The listing builds one solid part. Answer for the finished solid, in the listing's coordinates (mm). A direction names the side the tool comes from. Give positions to 0.01 mm unless a question says otherwise; leave off trailing zeros. Order: outer loops, then holes, each group sorted by start corner. A loop starts at its lowest first (then second) coordinate and runs counter-clockwise, first axis right, second up.
```python
from build123d import *

# Parameters (mm, degrees)
SKETCH_1_W          = 72
SKETCH_1_H          = 60
SKETCH_1_R          = 1.65
SKETCH_1_W_2        = 56
SKETCH_1_H_2        = 44
EXTRUDE_1_DEPTH     = 3
FILLET_1_R          = 3
SKETCH_2_R          = 1.65
EXTRUDE_2_DEPTH     = 3
FILLET_2_R          = 5
FILLET_3_R          = 6
SKETCH_3_W          = 6
SKETCH_3_H          = 20
CUT_EXTRUDE_1_DEPTH = 4
FILLET_4_R          = 2


with BuildPart() as part:
    # 草图1 → 凸台-拉伸1 (new body)
    with BuildSketch(Plane.XY):
        Rectangle(SKETCH_1_W, SKETCH_1_H)
        with Locations((31, -25)):
            Circle(SKETCH_1_R, mode=Mode.SUBTRACT)
        with Locations((31, 25)):
            Circle(SKETCH_1_R, mode=Mode.SUBTRACT)
        with Locations((-31, 25)):
            Circle(SKETCH_1_R, mode=Mode.SUBTRACT)
        with Locations((-31, -25)):
            Circle(SKETCH_1_R, mode=Mode.SUBTRACT)
        Rectangle(SKETCH_1_W_2, SKETCH_1_H_2, mode=Mode.SUBTRACT)
    extrude(amount=EXTRUDE_1_DEPTH)

    # 圆角1
    fillet_1_edges = [part.edges().sort_by_distance(p)[0] for p in [
        (-28, 22, 1.5),
        (-28, -22, 1.5),
        (28, -22, 1.5),
        (28, 22, 1.5),
    ]]
    fillet(fillet_1_edges, radius=FILLET_1_R)

    # 草图2 → 凸台-拉伸2 (add)
    with BuildSketch(Plane.XY.offset(3)):
        with BuildLine():
            Line((-46.723391823, 62.294305745), (-24.110675499, 30))
            Line((-24.110675499, 30), (-36, 30))
            Line((-36, 30), (-36, 20.51209678))
            Line((-36, 20.51209678), (-53.625231148, 58.309526953))
            ThreePointArc((-53.625231148, 58.309526953), (-52, 63.464101615), (-46.723391823, 62.294305745))
        make_face()
        with Locations((-50, 60)):
            Circle(SKETCH_2_R, mode=Mode.SUBTRACT)
        with BuildLine():
            Line((-46.723391823, -62.294305745), (-24.110675499, -30))
            Line((-24.110675499, -30), (-36, -30))
            Line((-36, -30), (-36, -20.51209678))
            Line((-36, -20.51209678), (-53.625231148, -58.309526953))
            ThreePointArc((-53.625231148, -58.309526953), (-52, -63.464101615), (-46.723391823, -62.294305745))
        make_face()
        with Locations((-50, -60)):
            Circle(SKETCH_2_R, mode=Mode.SUBTRACT)
        with BuildLine():
            Line((31.136296695, 61.03527618), (22.820419505, 30))
            Line((22.820419505, 30), (36, 30))
            Line((36, 30), (38.979882295, 59.59932941))
            ThreePointArc((38.979882295, 59.59932941), (35.720319493, 63.934607964), (31.136296695, 61.03527618))
        make_face()
        with Locations((35, 60)):
            Circle(SKETCH_2_R, mode=Mode.SUBTRACT)
        with BuildLine():
            Line((38.979882295, -59.59932941), (36, -30))
            Line((36, -30), (22.820419505, -30))
            Line((22.820419505, -30), (31.136296695, -61.03527618))
            ThreePointArc((31.136296695, -61.03527618), (35.720319493, -63.934607964), (38.979882295, -59.59932941))
        make_face()
        with Locations((35, -60)):
            Circle(SKETCH_2_R, mode=Mode.SUBTRACT)
    extrude(amount=-EXTRUDE_2_DEPTH)

    # 圆角2
    fillet_2_edges = [part.edges().sort_by_distance(p)[0] for p in [
        (22.820419505, -30, 1.5),
        (22.820419505, 30, 1.5),
        (-24.110675499, 30, 1.5),
        (36, 30, 1.5),
        (36, -30, 1.5),
        (-24.110675499, -30, 1.5),
    ]]
    fillet(fillet_2_edges, radius=FILLET_2_R)

    # 圆角3
    fillet_3_edges = [part.edges().sort_by_distance(p)[0] for p in [
        (-36, 20.51209678, 1.5),
        (-36, -20.51209678, 1.5),
    ]]
    fillet(fillet_3_edges, radius=FILLET_3_R)

    # 草图3 → 切除-拉伸1 (cut, through all)
    with BuildSketch(Plane.XY.offset(3)):
        with Locations((36, 0)):
            Rectangle(SKETCH_3_W, SKETCH_3_H)
    extrude(amount=-CUT_EXTRUDE_1_DEPTH, mode=Mode.SUBTRACT)

    # 圆角4
    fillet_4_edges = [part.edges().sort_by_distance(p)[0] for p in [
        (33, 10, 1.5),
        (33, -10, 1.5),
    ]]
    fillet(fillet_4_edges, radius=FILLET_4_R)


solid = part.part
```
1) Straight lines are drawn through the part: probe 1 along Y at (x, z) = (35, 1.4); probe 2 along X at (y, z) = (-14.5, 0.7); probe 3 along Y at (x, z) = (15, 2.7). For each, find the intervals that lie inside material, in ascending order.
Geometry says:
probe 1: y = -64 to -61.65, -58.35 to -10, 10 to 58.35, 61.65 to 64
probe 2: x = -36 to -28, 28 to 36
probe 3: y = -30 to -22, 22 to 30
2) Find section D-D (y = -47.5). Write down the section's boundary in (x, z), then the cut area to 3 significant figures.
Geometry says:
outline: (-48.58, 0) - (-36.36, 0) - (-36.36, 3) - (-48.58, 3) - close; (27.51, 0) - (37.76, 0) - (37.76, 3) - (27.51, 3) - close
area: 67.4 mm2
3) Given P1, Ø1.5, axis at y = -1, z = 1, coming from the +X side; P2, Ø0.9, axis at y = 3, z = 1.5, coming from the -X side; P3, Ø1.5, axis at y = 51, z = 1, coming from the +X side; P4, Ø2.5, axis at x = 31, y = -25, coming from the -Z side, each flat-ended and moving along its own axis, determine where each tip first touches the part or whether it passes through.
Geometry says:
P1: stops at x = 33
P2: stops at x = -36
P3: stops at x = 38.19
P4: passes through
4) A tool of negligible diameter and unlimited length cuts with its end or side. For faces 1 (the flat face through (-7, 24, 3)), 2 (the cylindrical face through (-27.1, -21.14, 1.52)), 3 (the flat face through (-2, -30, 1)), 4 (the flat face through (-36, 0, 1)), 5 (the flat face through (-7, 24, 0)), from which of +Z, -Z, +X, -X, +Y, -Y can it reach the whole face along a straight path? Write none if from no direction.
Geometry says:
face 1: +Z, +X, -X, +Y, -Y
face 2: +Z, -Z
face 3: +Z, -Z, -Y
face 4: +Z, -Z, -X
face 5: -Z, +X, -X, +Y, -Y
5) Find section B-B (y = 25). Write down the section's boundary in (x, z).
Geometry says:
outline: (-38.09, 0) - (-32.65, 0) - (-32.65, 3) - (-38.09, 3) - close; (-29.35, 0) - (29.35, 0) - (29.35, 3) - (-29.35, 3) - close; (32.65, 0) - (36, 0) - (36, 3) - (32.65, 3) - close
6) Find section C-C (x = -31). Write down the section's boundary in (y, z).
Geometry says:
outline: (-39.84, 0) - (-26.65, 0) - (-26.65, 3) - (-39.84, 3) - close; (-23.35, 0) - (23.35, 0) - (23.35, 3) - (-23.35, 3) - close; (26.65, 0) - (39.84, 0) - (39.84, 3) - (26.65, 3) - close
7) For a pull along X with two mould halves and no side action, classify faces 6 (the cylindrical face through (27.1, -21.14, 1.52)), 7 (the cylindrical face through (-52.072, 63.422, 1.521)), 8 (the flat face through (36, -20, 1)), 9 (the flat face through (-44.974, -39.757, 1.521)) as +X half, -X half, draft (parallel to the pull), parting line (faces both ways), or undercut.
Geometry says:
face 6: undercut
face 7: undercut
face 8: +X half
face 9: -X half
8) Find section A-A (x = 11.5). Write down the section's boundary in (y, z).
Geometry says:
outline: (-30, 0) - (-22, 0) - (-22, 3) - (-30, 3) - close; (22, 0) - (30, 0) - (30, 3) - (22, 3) - close
